from build123d import *

# Parameters (mm, degrees)
F3_DEPTH  = 5.08
F5_W      = 7.62
F5_H      = 5.08
F6_DEPTH  = 38.101
F8_W      = 7.62
F8_H      = 5.08
F9_DEPTH  = 25.401
F10_R     = 1.905
F10_W     = 7.62
F10_H     = 2.54
F11_DEPTH = 12.7
F12_R     = 5.08


with BuildPart() as f1:
    # F0 (on Front) → F1 (revolve)
    with BuildSketch(Plane.XZ):
        Polygon((12.7, 50.8), (12.7, 0), (25.4, 0), (19.05, 31.75), (25.4, 50.8), align=None)
    revolve(axis=Axis((12.7, 0, 25.4), (0, 0, -1)))

    # F2 (on face) → F3 (join)
    with BuildSketch(Plane.XY.offset(50.8)):
        with BuildLine():
            ThreePointArc((0, 0), (3.7197438789, -8.9802561211), (12.7, -12.7))
            Line((12.7, -12.7), (12.7, -8.9802561211))
            Line((12.7, -8.9802561211), (12.6097438789, -8.9802561211))
            ThreePointArc((12.6097438789, -8.9802561211), (6.3235645942, -6.3764354058), (3.7197438789, -0.0902561211))
            Line((3.7197438789, -0.0902561211), (3.7197438789, 0.0902561211))
            ThreePointArc((3.7197438789, 0.0902561211), (6.3235645942, 6.3764354058), (12.6097438789, 8.9802561211))
            Line((12.6097438789, 8.9802561211), (12.7, 8.9802561211))
            Line((12.7, 8.9802561211), (12.7, 12.7))
            ThreePointArc((12.7, 12.7), (3.7197438789, 8.9802561211), (0, 0))
        make_face()
        with BuildLine():
            Line((12.7, -8.9802561211), (12.7, -12.7))
            ThreePointArc((12.7, -12.7), (21.6802561211, -8.9802561211), (25.4, 0))
            ThreePointArc((25.4, 0), (21.6802561211, 8.9802561211), (12.7, 12.7))
            Line((12.7, 12.7), (12.7, 8.9802561211))
            Line((12.7, 8.9802561211), (12.7902561211, 8.9802561211))
            ThreePointArc((12.7902561211, 8.9802561211), (19.0764354058, 6.3764354058), (21.6802561211, 0.0902561211))
            Line((21.6802561211, 0.0902561211), (21.6802561211, -0.0902561211))
            ThreePointArc((21.6802561211, -0.0902561211), (19.0764354058, -6.3764354058), (12.7902561211, -8.9802561211))
            Line((12.7902561211, -8.9802561211), (12.7, -8.9802561211))
        make_face()
    extrude(amount=F3_DEPTH)

    # F5 (on offset) → F6 (cut, through all)
    with BuildSketch(Plane.XZ.offset(25.4)):
        with Locations((12.6097438789, 53.34)):
            Rectangle(F5_W, F5_H)
    extrude(amount=-F6_DEPTH, mode=Mode.SUBTRACT)

    # F8 (on offset) → F9 (cut, through all)
    with BuildSketch(Plane.YZ.offset(25.4)):
        with Locations((0, 53.34)):
            Rectangle(F8_W, F8_H)
    extrude(amount=-F9_DEPTH, mode=Mode.SUBTRACT)

    # F10 (on Front) → F11 (join)
    with BuildSketch(Plane.XZ):
        with Locations((7.5297438789, 46.99)):
            Circle(F10_R)
        with Locations((17.6897438789, 46.99)):
            Circle(F10_R)
        with Locations((12.6097438789, 43.18)):
            Rectangle(F10_W, F10_H)
    extrude(amount=F11_DEPTH)

    # F12
    f12_edges = [f1.edges().sort_by_distance(p)[0] for p in [
        (6.35, 0, 31.75),
    ]]
    fillet(f12_edges, radius=F12_R)


solid = f1.part
Work out the finished part from the listing and answer in its coordinate system (mm). A direction names the side the tool comes from. Give positions to 0.01 mm unless a question says otherwise; leave off trailing zeros. Order: outer loops, then holes, each group sorted by start corner. A loop starts at its lowest first (then second) coordinate and runs counter-clockwise, first axis right, second up. Notation, with made-up numbers: (-30, 51.25) -> (9, 51.25) arc R16 cw to (9, 55.25) -> close; hole circle Ø6 at (84.5, -18.5). An arc over 180 degrees is marked (long way). One line per item, written item: value.
Item 1: Find section A-A, the plane z = 12. Give the vertices of the cut face in (x, y).
Answer sheet:
outline: circle Ø20.6 at (12.7, 0)
Item 2: Find section B-B, the plane z = 46.99. Give the vertices of the cut face in (x, y), plus the area to 3 significant figures.
Answer sheet:
outline: (5.62, -12.7) -> (9.43, -12.7) -> (9.43, -10.95) arc R11.43 ccw to (15.78, -11.01) -> (15.78, -12.7) -> (19.59, -12.7) -> (19.59, -9.12) arc R11.43 ccw (long way) to (5.62, -8.98) -> close
area: 430 mm²
Item 3: A tool of negligible diameter and unlimited length cuts with its end or side. For faces 4 (the flat face through (3, 3.81, 53)), 5 (the flat face through (8.8, 10, 53)), 6 (the cylindrical face through (6.26, 6.31, 53.3)), 7 (the conical face through (10.723, 8.905, 40.065)), from which of +Z, -Z, +X, -X, +Y, -Y can it reach the whole face along a straight path? Write none if from no direction.
Answer sheet:
face 4: +Z, +X, -X
face 5: +Z, +Y, -Y
face 6: +Z
face 7: none
Item 4: Find section C-C, the plane z = 22. Give the vertices of the cut face in (x, y).
Answer sheet:
outline: circle Ø16.6 at (12.7, 0)
Item 5: Straight lines are drawn through the part: probe 1 along X at (y, z) = (-10.75, 51); probe 2 along Z at (x, y) = (14.75, 2); probe 3 along Y at (x, z) = (2.5, 52). For each, find the intervals that lie inside material, in ascending order.
Answer sheet:
probe 1: 5.94 to 8.8, 16.42 to 19.46
probe 2: 0 to 50.8
probe 3: -7.57 to -3.81, 3.81 to 7.57
Item 6: Determine the mould class of faces 1 (the flat face through (8.8, -11, 43)), 2 (the flat face through (13, 0, 0)), 3 (the cylindrical face through (19.45, -11.2, 46.26)) for opening direction X: released by +X, released by -X, zero draft, split by the parting line, or undercut.
Answer sheet:
face 1: released by -X
face 2: zero draft
face 3: undercut
Item 7: Flat-ended cylindrical pins translate along their axes: P1, Ø1.2, axis at x = 22, z = 52.5, coming from the +Y side; P2, Ø3, axis at y = -11, z = 53, coming from the +X side; P3, Ø4.5, axis at x = 24, z = 54, coming from the -Y side. Find the tip coordinate at first contact, or state that the pin passes through.
Answer sheet:
P1: y = 9.25
P2: x = 21.13
P3: y = -8.91
